The model under review builds one solid part; all positions refer to its coordinate system, in mm. Coordinates: 2 decimals unless noted, no trailing zeros. Loops run counter-clockwise (first coordinate to the right, second up) from the corner with the lowest first, then second, coordinate; pieces in that order, holes last. Notation, with made-up numbers: (23, -2.5) - (65, -2.5) arc R14 ccw to (65, 10.5) - close; hole circle Ø6 at (34.25, 82). An arc over 180 degrees is marked (long way). Answer in a Markdown table with one row per item. Add a question column.
(1) We need section B-B on z = -250. Write out the cut boundary in (x, y), plus the area to 3 significant figures.
(2) For line 1 along X through (y, z) = (6.5, -234.6); line 2 along Z through (x, y) = (375, 2); line 3 along X through (y, z) = (5.75, -350), list the stretches that pass through material, from the lowest coordinate up.
(3) We need section A-A on x = 45. Write out the cut boundary in (y, z), plus the area to 3 significant figures.
(4) For P1, Ø4, axis at x = 125, z = -350, coming from the +Y side; P2, Ø4, axis at x = 470.4, z = -234.6, coming from the +Y side, all flat-tipped, find the tip position at first contact; note any pin that passes through.
from build123d import *

# Parameters (mm, degrees)
SZKIC1_W                                             = 500
SZKIC1_H                                             = 500
DODANIE_WYCI_GNI_CIE1_DEPTH                          = 10
SZKIC2_R                                             = 12.5
WYTNIJ_WYCI_GNI_CIE1_DEPTH                           = 708.177488329
POG_BIENIE_STO_KOWE_POD_M3_WKR_T_USTALAJ_D           = 3.4
POG_BIENIE_STO_KOWE_POD_M3_WKR_T_USTALAJ_CSINK_D     = 6.72
POG_BIENIE_STO_KOWE_POD_M3_WKR_T_USTALAJ_CSINK_ANGLE = 90
POG_BIENIE_STO_KOWE_POD_M3_WKR_T_DO_CZ_C_D           = 3.4
POG_BIENIE_STO_KOWE_POD_M3_WKR_T_DO_CZ_C_DEPTH       = 10
POG_BIENIE_STO_KOWE_POD_M3_WKR_T_DO_CZ_C_CSINK_D     = 6.3
POG_BIENIE_STO_KOWE_POD_M3_WKR_T_DO_CZ_C_CSINK_ANGLE = 90
POG_BIENIE_STO_KOWE_POD_M3_WKR_T_DO_CZ_C_TIP         = 1.021463052
OTWORY_USTALAJ_CE_3_0MM1_D                           = 3
OTWORY_USTALAJ_CE_3_0MM1_DEPTH                       = 10
OTWORY_USTALAJ_CE_3_0MM1_TIP                         = 0.901290929
OTWORY_USTALAJ_CE_3_0MM2_D                           = 3
OTWORY_USTALAJ_CE_3_0MM2_DEPTH                       = 10
OTWORY_USTALAJ_CE_3_0MM2_TIP                         = 0.901290929


with BuildPart() as part:
    # Szkic1 → Dodanie-wyciągnięcie1 (new body)
    with BuildSketch(Plane(origin=(0, 0, 0), x_dir=(1, 0, 0), z_dir=(0, 1, 0))):
        with Locations((250, 250)):
            Rectangle(SZKIC1_W, SZKIC1_H)
    extrude(amount=DODANIE_WYCI_GNI_CIE1_DEPTH)

    # Szkic2 → Wytnij-wyciągnięcie1 (cut, through all)
    with BuildSketch(Plane(origin=(0, 10, 0), x_dir=(1, 0, 0), z_dir=(0, 1, 0))):
        with Locations(Location((45, 250, 0), (0, 0, 270))):
            Circle(SZKIC2_R)
        with Locations(Location((455, 250, 0), (0, 0, 270))):
            Circle(SZKIC2_R)
    extrude(amount=-WYTNIJ_WYCI_GNI_CIE1_DEPTH, mode=Mode.SUBTRACT)

    # Pogłębienie stożkowe pod M3 Wkręt ustalający1 (through all)
    with Locations(Plane(origin=(0, 10, 0), x_dir=(1, 0, 0), z_dir=(0, 1, 0))):
        with Locations((439.6, 265.4), (439.6, 234.6), (470.4, 234.6), (470.4, 265.4), (60.4, 234.6), (60.4, 265.4), (29.6, 234.6), (29.6, 265.4)):
            CounterSinkHole(POG_BIENIE_STO_KOWE_POD_M3_WKR_T_USTALAJ_D / 2, POG_BIENIE_STO_KOWE_POD_M3_WKR_T_USTALAJ_CSINK_D / 2, counter_sink_angle=POG_BIENIE_STO_KOWE_POD_M3_WKR_T_USTALAJ_CSINK_ANGLE)

    # Pogłębienie stożkowe pod M3 wkręt do części metalowych z łbem soczewkowym1
    with Locations(Plane(origin=(0, 10, 0), x_dir=(1, 0, 0), z_dir=(0, 1, 0))):
        with Locations((375, 350), (375, 150), (125, 350), (125, 150)):
            CounterSinkHole(POG_BIENIE_STO_KOWE_POD_M3_WKR_T_DO_CZ_C_D / 2, POG_BIENIE_STO_KOWE_POD_M3_WKR_T_DO_CZ_C_CSINK_D / 2, depth=POG_BIENIE_STO_KOWE_POD_M3_WKR_T_DO_CZ_C_DEPTH, counter_sink_angle=POG_BIENIE_STO_KOWE_POD_M3_WKR_T_DO_CZ_C_CSINK_ANGLE)
            with Locations((0, 0, -(POG_BIENIE_STO_KOWE_POD_M3_WKR_T_DO_CZ_C_DEPTH + POG_BIENIE_STO_KOWE_POD_M3_WKR_T_DO_CZ_C_TIP / 2))):  # 118° drill point
                Cone(0, POG_BIENIE_STO_KOWE_POD_M3_WKR_T_DO_CZ_C_D / 2, POG_BIENIE_STO_KOWE_POD_M3_WKR_T_DO_CZ_C_TIP, mode=Mode.SUBTRACT)

    # Otwory ustalające Ø3.0mm1
    with Locations(Plane(origin=(0, 0, 0), x_dir=(-1, 0, 0), z_dir=(0, -1, 0))):
        with Locations((-486, 490), (-486, 10), (-14, 10), (-14, 490)):
            Hole(OTWORY_USTALAJ_CE_3_0MM1_D / 2, depth=OTWORY_USTALAJ_CE_3_0MM1_DEPTH)
            with Locations((0, 0, -(OTWORY_USTALAJ_CE_3_0MM1_DEPTH + OTWORY_USTALAJ_CE_3_0MM1_TIP / 2))):  # 118° drill point
                Cone(0, OTWORY_USTALAJ_CE_3_0MM1_D / 2, OTWORY_USTALAJ_CE_3_0MM1_TIP, mode=Mode.SUBTRACT)

    # Otwory ustalające Ø3.0mm2
    with Locations(Plane(origin=(0, 0, 0), x_dir=(-1, 0, 0), z_dir=(0, -1, 0))):
        with Locations((-150, 495), (-350, 495)):
            Hole(OTWORY_USTALAJ_CE_3_0MM2_D / 2, depth=OTWORY_USTALAJ_CE_3_0MM2_DEPTH)
            with Locations((0, 0, -(OTWORY_USTALAJ_CE_3_0MM2_DEPTH + OTWORY_USTALAJ_CE_3_0MM2_TIP / 2))):  # 118° drill point
                Cone(0, OTWORY_USTALAJ_CE_3_0MM2_D / 2, OTWORY_USTALAJ_CE_3_0MM2_TIP, mode=Mode.SUBTRACT)


solid = part.part
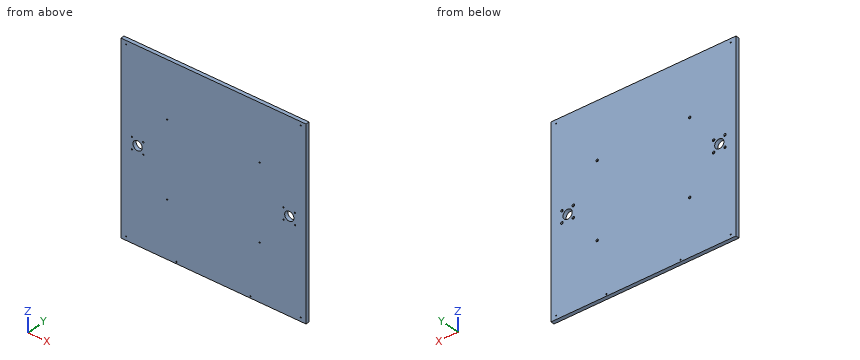
Outcome:
| question | item | result |
|---|---|---|
| 1 | outline | (0, 0) - (32.5, 0) - (32.5, 10) - (0, 10) - close; (57.5, 0) - (442.5, 0) - (442.5, 10) - (57.5, 10) - close; (467.5, 0) - (500, 0) - (500, 10) - (467.5, 10) - close |
| 1 | area | 4,500 mm² |
| 2 | line 1 | 0 to 27.9, 31.3 to 58.7, 62.1 to 437.9, 441.3 to 468.7, 472.1 to 500 |
| 2 | line 2 | -500 to -351.7, -348.3 to -151.7, -148.3 to 0 |
| 2 | line 3 | 0 to 123.3, 126.7 to 373.3, 376.7 to 500 |
| 3 | outline | (0, -500) - (10, -500) - (10, -262.5) - (0, -262.5) - close; (0, -237.5) - (10, -237.5) - (10, 0) - (0, 0) - close |
| 3 | area | 4,750 mm² |
| 4 | P1 | y = 8.85 |
| 4 | P2 | y = 8.64 |
